Check sheet for the modelled part. Datum: model origin and axes. Units: mm. A direction names the side the tool comes from. Give positions to 0.01 mm unless a question says otherwise; leave off trailing zeros. Order: outer loops, then holes, each group sorted by start corner. A loop starts at its lowest first (then second) coordinate and runs counter-clockwise, first axis right, second up.
Item 1: Gauge pin test, flat ends, axial feed: P1, Ø5, axis at x = -132, z = -6.5, coming from the +Y side; P2, Ø2, axis at x = -120, y = 118.5, coming from the -Z side; P3, Ø3, axis at x = -170, z = -6.5, coming from the +Y side. Record the tip position at first contact, or that the pin passes through.
Item 2: Sectioned sample at C-C on x = -201. Record the boundary of the cut face in (y, z), and give its area (3 significant figures).
Item 3: Material ranges on line 1 along Y through (x, z) = (-190.5, 6.25); line 2 along X through (y, z) = (90.5, 8); line 3 along Y through (x, z) = (-109.5, 3.25), recorded low to high.
Item 4: Sectioned sample at A-A on y = 111.5. Record the boundary of the cut face in (x, z), and give its area (3 significant figures).
Item 5: Release check for a two-part mould opening along X. For faces 1 (the flat face through (-91, 82, -10)), 2 (the flat face through (-85.849, 100, 5)), 3 (the flat face through (-173.849, 85, -3)), 4 (the flat face through (-111, 83, 7)) record: released by +X, released by -X, zero draft, split by the parting line, or undercut.
Item 6: Access from +Z, -Z, +X, -X, +Y, -Y to the whole of each face (thin tool, end or side, straight path). Record for faces 5 (the flat face through (-127, 87, -5)), 6 (the flat face through (-111, 99, 7)), 7 (the flat face through (-148, 115, 5)).
Item 7: Sectioned sample at B-B on z = 6.5. Record the boundary of the cut face in (x, y).
Item 8: Sectioned sample at D-D on y = 96.5. Record the boundary of the cut face in (x, z), and give its area (3 significant figures).
from build123d import *

# Parameters (mm, degrees)
SKETCH1_W               = 130
SKETCH1_H               = 50
BOSS_EXTRUDE1_DEPTH     = 15
CUT_EXTRUDE1_DEPTH      = 1
CUT_EXTRUDE1_DEPTH_BACK = 127
SKETCH4_W               = 10
SKETCH4_H               = 3
BOSS_EXTRUDE2_DEPTH     = 10
SKETCH6_W               = 30
SKETCH6_H               = 16
CUT_EXTRUDE2_DEPTH      = 16
SKETCH7_R               = 1.375
CUT_EXTRUDE3_DEPTH      = 4
SKETCH9_W               = 10
SKETCH9_H               = 3
BOSS_EXTRUDE4_DEPTH     = 10
SKETCH10_R              = 1.375
CUT_EXTRUDE4_DEPTH      = 10
SKETCH11_W              = 10
SKETCH11_H              = 1
BOSS_EXTRUDE5_DEPTH     = 20
SKETCH13_W              = 10
SKETCH13_H              = 3
CUT_EXTRUDE5_DEPTH      = 10
SKETCH14_W              = 10
SKETCH14_H              = 3
CUT_EXTRUDE6_DEPTH      = 10
SKETCH15_W              = 10
SKETCH15_H              = 3
CUT_EXTRUDE7_DEPTH      = 10
SKETCH16_W              = 10
SKETCH16_H              = 3
BOSS_EXTRUDE6_DEPTH     = 10
BOSS_EXTRUDE8_DEPTH     = 10
BOSS_EXTRUDE9_DEPTH     = 10
BOSS_EXTRUDE10_DEPTH    = 10
BOSS_EXTRUDE11_DEPTH    = 10
SKETCH29_W              = 6
SKETCH29_H              = 10
CUT_EXTRUDE10_DEPTH     = 10
SKETCH30_W              = 6
SKETCH30_H              = 10
CUT_EXTRUDE11_DEPTH     = 10
SKETCH31_W              = 6
SKETCH31_H              = 10
CUT_EXTRUDE12_DEPTH     = 10
SKETCH32_W              = 6
SKETCH32_H              = 10
CUT_EXTRUDE13_DEPTH     = 10
SKETCH35_R              = 1.4
CUT_EXTRUDE14_DEPTH     = 5


with BuildPart() as part:
    # Sketch1 → Boss-Extrude1 (new body)
    with BuildSketch(Plane.XY):
        with Locations((-150.849056604, 105)):
            Rectangle(SKETCH1_W, SKETCH1_H)
    extrude(amount=BOSS_EXTRUDE1_DEPTH)

    # Sketch3 → Cut-Extrude1 (cut, two sides)
    with BuildSketch(Plane(origin=(-85.849056604, 0, 0), x_dir=(0, 0, -1), z_dir=(1, 0, 0))) as cut_extrude1_sk:
        Polygon((-14, 125), (-5, 125), (-5, 105), (-14, 105), (-14, 107), (-15, 107), (-15, 123), (-14, 123), align=None)
    extrude(amount=CUT_EXTRUDE1_DEPTH, mode=Mode.SUBTRACT)
    extrude(cut_extrude1_sk.sketch, amount=-CUT_EXTRUDE1_DEPTH_BACK, mode=Mode.SUBTRACT)

    # Sketch4 → Boss-Extrude2 (add)
    with BuildSketch(Plane(origin=(0, 0, 0), x_dir=(-1, 0, 0), z_dir=(0, 0, -1))):
        with Locations((105.849056604, 81.5)):
            Rectangle(SKETCH4_W, SKETCH4_H)
        with Locations((195.849056604, 81.5)):
            Rectangle(SKETCH4_W, SKETCH4_H)
    extrude(amount=BOSS_EXTRUDE2_DEPTH)

    # Sketch6 → Cut-Extrude2 (cut, through all)
    with BuildSketch(Plane(origin=(0, 0, 0), x_dir=(-1, 0, 0), z_dir=(0, 0, -1))):
        with Locations((190.849056604, 91)):
            Rectangle(SKETCH6_W, SKETCH6_H)
        with Locations((150.849056604, 91)):
            Rectangle(SKETCH6_W, SKETCH6_H)
        with Locations((110.849056604, 91)):
            Rectangle(SKETCH6_W, SKETCH6_H)
    extrude(amount=-CUT_EXTRUDE2_DEPTH, mode=Mode.SUBTRACT)

    # Sketch7 → Cut-Extrude3 (cut, through all)
    with BuildSketch(Plane(origin=(0, 83, 0), x_dir=(1, 0, 0), z_dir=(0, 1, 0))):
        with Locations((-105.849056604, 5)):
            Circle(SKETCH7_R)
    cut_extrude3 = extrude(amount=-CUT_EXTRUDE3_DEPTH, mode=Mode.SUBTRACT)

    # Mirror1: Cut-Extrude3 across plane
    add(cut_extrude3.mirror(Plane(origin=(-151, 0, 0), x_dir=(0, 0, 1), z_dir=(1, 0, 0))), mode=Mode.SUBTRACT)

    # Sketch9 → Boss-Extrude4 (add)
    with BuildSketch(Plane(origin=(0, 0, 0), x_dir=(-1, 0, 0), z_dir=(0, 0, -1))):
        with Locations((150.849056604, 81.5)):
            Rectangle(SKETCH9_W, SKETCH9_H)
    extrude(amount=BOSS_EXTRUDE4_DEPTH)

    # Sketch10 → Cut-Extrude4 (cut)
    with BuildSketch(Plane(origin=(0, 83, 0), x_dir=(1, 0, 0), z_dir=(0, 1, 0))):
        with Locations((-150.849056604, 5)):
            Circle(SKETCH10_R)
    extrude(amount=-CUT_EXTRUDE4_DEPTH, mode=Mode.SUBTRACT)

    # Sketch11 → Boss-Extrude5 (add)
    with BuildSketch(Plane(origin=(0, 107, 0), x_dir=(1, 0, 0), z_dir=(0, 1, 0))):
        with Locations((-90.849056604, -14.5)):
            Rectangle(SKETCH11_W, SKETCH11_H)
    extrude(amount=BOSS_EXTRUDE5_DEPTH)

    # Sketch13 → Cut-Extrude5 (cut)
    with BuildSketch(Plane(origin=(0, 0, -10), x_dir=(-1, 0, 0), z_dir=(0, 0, -1))):
        with Locations((105.849056604, 81.5)):
            Rectangle(SKETCH13_W, SKETCH13_H)
    extrude(amount=-CUT_EXTRUDE5_DEPTH, mode=Mode.SUBTRACT)

    # Sketch14 → Cut-Extrude6 (cut)
    with BuildSketch(Plane(origin=(0, 0, -10), x_dir=(-1, 0, 0), z_dir=(0, 0, -1))):
        with Locations((150.849056604, 81.5)):
            Rectangle(SKETCH14_W, SKETCH14_H)
    extrude(amount=-CUT_EXTRUDE6_DEPTH, mode=Mode.SUBTRACT)

    # Sketch15 → Cut-Extrude7 (cut)
    with BuildSketch(Plane(origin=(0, 0, -10), x_dir=(-1, 0, 0), z_dir=(0, 0, -1))):
        with Locations((195.849056604, 81.5)):
            Rectangle(SKETCH15_W, SKETCH15_H)
    extrude(amount=-CUT_EXTRUDE7_DEPTH, mode=Mode.SUBTRACT)

    # Sketch16 → Boss-Extrude6 (add)
    with BuildSketch(Plane(origin=(0, 0, 0), x_dir=(-1, 0, 0), z_dir=(0, 0, -1))):
        with Locations((90.849056604, 81.5)):
            Rectangle(SKETCH16_W, SKETCH16_H)
        with Locations((130.849056604, 81.5)):
            Rectangle(SKETCH16_W, SKETCH16_H)
        with Locations((170.849056604, 81.5)):
            Rectangle(SKETCH16_W, SKETCH16_H)
        with Locations((210.849056604, 81.5)):
            Rectangle(SKETCH16_W, SKETCH16_H)
    extrude(amount=BOSS_EXTRUDE6_DEPTH)

    # Sketch18 → Boss-Extrude8 (add)
    with BuildSketch(Plane(origin=(-85.849056604, 0, 0), x_dir=(0, 0, -1), z_dir=(1, 0, 0))):
        Polygon((10, 83), (0, 91.236285037), (0, 83), align=None)
    extrude(amount=-BOSS_EXTRUDE8_DEPTH)

    # Sketch20 → Boss-Extrude9 (add)
    with BuildSketch(Plane(origin=(-125.849056604, 0, 0), x_dir=(0, 0, -1), z_dir=(1, 0, 0))):
        Polygon((0, 83), (0, 91), (10, 83), align=None)
    extrude(amount=-BOSS_EXTRUDE9_DEPTH)

    # Sketch21 → Boss-Extrude10 (add)
    with BuildSketch(Plane(origin=(-165.849056604, 0, 0), x_dir=(0, 0, -1), z_dir=(1, 0, 0))):
        Polygon((0, 83), (0, 91), (10, 83), align=None)
    extrude(amount=-BOSS_EXTRUDE10_DEPTH)

    # Sketch22 → Boss-Extrude11 (add)
    with BuildSketch(Plane(origin=(-205.849056604, 0, 0), x_dir=(0, 0, -1), z_dir=(1, 0, 0))):
        Polygon((0, 83), (0, 91), (10, 83), align=None)
    extrude(amount=-BOSS_EXTRUDE11_DEPTH)

    # Sketch29 → Cut-Extrude10 (cut)
    with BuildSketch(Plane(origin=(0, 0, -10), x_dir=(-1, 0, 0), z_dir=(0, 0, -1))):
        with Locations((90.849056604, 88)):
            Rectangle(SKETCH29_W, SKETCH29_H)
    extrude(amount=-CUT_EXTRUDE10_DEPTH, mode=Mode.SUBTRACT)

    # Sketch30 → Cut-Extrude11 (cut)
    with BuildSketch(Plane(origin=(0, 0, -10), x_dir=(-1, 0, 0), z_dir=(0, 0, -1))):
        with Locations((130.849056604, 88)):
            Rectangle(SKETCH30_W, SKETCH30_H)
    extrude(amount=-CUT_EXTRUDE11_DEPTH, mode=Mode.SUBTRACT)

    # Sketch31 → Cut-Extrude12 (cut)
    with BuildSketch(Plane(origin=(0, 0, -10), x_dir=(-1, 0, 0), z_dir=(0, 0, -1))):
        with Locations((170.849056604, 88)):
            Rectangle(SKETCH31_W, SKETCH31_H)
    extrude(amount=-CUT_EXTRUDE12_DEPTH, mode=Mode.SUBTRACT)

    # Sketch32 → Cut-Extrude13 (cut)
    with BuildSketch(Plane(origin=(0, 0, -10), x_dir=(-1, 0, 0), z_dir=(0, 0, -1))):
        with Locations((210.849056604, 88)):
            Rectangle(SKETCH32_W, SKETCH32_H)
    extrude(amount=-CUT_EXTRUDE13_DEPTH, mode=Mode.SUBTRACT)

    # Sketch35 → Cut-Extrude14 (cut)
    with BuildSketch(Plane(origin=(0, 83, 0), x_dir=(1, 0, 0), z_dir=(0, 1, 0))):
        with Locations((-210.849056604, 5)):
            Circle(SKETCH35_R)
        with Locations((-170.849056604, 5)):
            Circle(SKETCH35_R)
        with Locations((-130.849056604, 5)):
            Circle(SKETCH35_R)
        with Locations((-90.849056604, 5)):
            Circle(SKETCH35_R)
    extrude(amount=-CUT_EXTRUDE14_DEPTH, mode=Mode.SUBTRACT)


solid = part.part
Report:
1. P1: stops at y = 87.15
1. P2: stops at z = 0
1. P3: stops at y = 83
2. outline: (80, 0) - (83, 0) - (83, 15) - (80, 15) - close; (99, 0) - (130, 0) - (130, 15) - (123, 15) - (123, 14) - (125, 14) - (125, 5) - (105, 5) - (105, 14) - (107, 14) - (107, 15) - (99, 15) - close
2. area: 314 mm2
3. line 1: y = 80 to 83, 99 to 105, 125 to 130
3. line 2: x = -215.85 to -205.85, -175.85 to -165.85, -135.85 to -125.85, -95.85 to -85.85
3. line 3: y = 80 to 83, 99 to 130
4. outline: (-215.85, 0) - (-85.85, 0) - (-85.85, 5) - (-212.85, 5) - (-212.85, 15) - (-215.85, 15) - close; (-95.85, 14) - (-85.85, 14) - (-85.85, 15) - (-95.85, 15) - close
4. area: 690 mm2
5. face 1: zero draft
5. face 2: released by +X
5. face 3: undercut
5. face 4: undercut
6. face 5: -Z, -X, +Y
6. face 6: +Z, -Z
6. face 7: +X
7. outline: (-215.85, 80) - (-85.85, 80) - (-85.85, 105) - (-212.85, 105) - (-212.85, 125) - (-85.85, 125) - (-85.85, 130) - (-215.85, 130) - close; hole (-205.85, 83) - (-175.85, 83) - (-175.85, 99) - (-205.85, 99) - close; hole (-165.85, 83) - (-135.85, 83) - (-135.85, 99) - (-165.85, 99) - close; hole (-125.85, 83) - (-95.85, 83) - (-95.85, 99) - (-125.85, 99) - close
8. outline: (-215.85, 0) - (-205.85, 0) - (-205.85, 15) - (-215.85, 15) - close; (-175.85, 0) - (-165.85, 0) - (-165.85, 15) - (-175.85, 15) - close; (-135.85, 0) - (-125.85, 0) - (-125.85, 15) - (-135.85, 15) - close; (-95.85, 0) - (-85.85, 0) - (-85.85, 15) - (-95.85, 15) - close
8. area: 600 mm2
